```python
from build123d import *

# Parameters (mm, degrees)
STRUCTURAL_MEMBER1_DEPTH       = 1447.8
SKETCH12_R                     = 20.6375
CUT_EXTRUDE1_DEPTH             = 1451.304412873
F_1_2_0_5_DIAMETER_HOLE1_D     = 12.7
F_1_2_0_5_DIAMETER_HOLE1_DEPTH = 25.4
F_1_2_0_5_DIAMETER_HOLE1_TIP   = 3.815464931


with BuildPart() as part:
    # Sketch11 → Structural Member1 (new body)
    with BuildSketch(Plane(origin=(0, 0, 0), x_dir=(0, -1, 0), z_dir=(-1, 0, 0))):
        with BuildLine():
            Line((-25.4, -38.1), (25.4, -38.1))
            ThreePointArc((25.4, -38.1), (34.380256121, -34.380256121), (38.1, -25.4))
            Line((38.1, -25.4), (38.1, 25.4))
            ThreePointArc((38.1, 25.4), (34.380256121, 34.380256121), (25.4, 38.1))
            Line((25.4, 38.1), (-25.4, 38.1))
            ThreePointArc((-25.4, 38.1), (-34.380256121, 34.380256121), (-38.1, 25.4))
            Line((-38.1, 25.4), (-38.1, -25.4))
            ThreePointArc((-38.1, -25.4), (-34.380256121, -34.380256121), (-25.4, -38.1))
        make_face()
        with BuildLine():
            Line((-25.4, -34.925), (25.4, -34.925))
            ThreePointArc((25.4, -34.925), (32.135192091, -32.135192091), (34.925, -25.4))
            Line((34.925, -25.4), (34.925, 25.4))
            ThreePointArc((34.925, 25.4), (32.135192091, 32.135192091), (25.4, 34.925))
            Line((25.4, 34.925), (-25.4, 34.925))
            ThreePointArc((-25.4, 34.925), (-32.135192091, 32.135192091), (-34.925, 25.4))
            Line((-34.925, 25.4), (-34.925, -25.4))
            ThreePointArc((-34.925, -25.4), (-32.135192091, -32.135192091), (-25.4, -34.925))
        make_face(mode=Mode.SUBTRACT)
    extrude(amount=STRUCTURAL_MEMBER1_DEPTH)

    # Sketch12 → Cut-Extrude1 (cut, through all)
    with BuildSketch(Plane(origin=(0, 38.1, 0), x_dir=(1, 0, 0), z_dir=(0, 1, 0))):
        with Locations(Location((-723.9, 0, 0), (0, 0, 180))):
            Circle(SKETCH12_R)
    extrude(amount=-CUT_EXTRUDE1_DEPTH, mode=Mode.SUBTRACT)

    # 1/2 (0.5) Diameter Hole1
    with Locations(Plane(origin=(-800.1, 38.1, 0), x_dir=(0, 0, 1), z_dir=(0, 1, 0))):
        with Locations((0, 0), (0, 152.4)):
            Hole(F_1_2_0_5_DIAMETER_HOLE1_D / 2, depth=F_1_2_0_5_DIAMETER_HOLE1_DEPTH)
            with Locations((0, 0, -(F_1_2_0_5_DIAMETER_HOLE1_DEPTH + F_1_2_0_5_DIAMETER_HOLE1_TIP / 2))):  # 118° drill point
                Cone(0, F_1_2_0_5_DIAMETER_HOLE1_D / 2, F_1_2_0_5_DIAMETER_HOLE1_TIP, mode=Mode.SUBTRACT)


solid = part.part
```
Part model, mm, in its own coordinate system. A direction names the side the tool comes from. Round coordinates to 2 decimals unless told otherwise and drop trailing zeros. Loops run counter-clockwise (first coordinate to the right, second up) from the corner with the lowest first, then second, coordinate; pieces in that order, holes last.
1. Two-plate mould, pull along X, no slides. Class faces 1 (the face through (-1447.8, 0, -37)), 2 (the face through (0, 0, -37)), 3 (the face through (-714, 34.925, -22)), 4 (the face through (-703.282, 36.535, 0.907)): pulls with the +X half, pulls with the -X half, needs draft (parallel to the pull), parting line crosses it, or undercut.
Solutions:
face 1: pulls with the -X half
face 2: pulls with the +X half
face 3: needs draft
face 4: undercut
2. Drill centre lines: line 1 along Y through (x, z) = (-253.5, 13.5) (3 decimals); line 2 along Y through (x, z) = (-817, 33.5). Where is each one in solid material? Low to high.
Solutions:
line 1: y = -38.1 to -34.925, 34.925 to 38.1
line 2: y = -35.18 to -30.41, 30.41 to 35.18
3. Slice it at C-C (x = -236). Give the cut face in (y, z) (3 decimals), and give its area (3 significant figures).
Solutions:
outline: (-38.1, -25.4) arc R12.7 ccw to (-25.4, -38.1) - (25.4, -38.1) arc R12.7 ccw to (38.1, -25.4) - (38.1, 25.4) arc R12.7 ccw to (25.4, 38.1) - (-25.4, 38.1) arc R12.7 ccw to (-38.1, 25.4) - close; hole (-34.925, -25.4) arc R9.525 ccw to (-25.4, -34.925) - (25.4, -34.925) arc R9.525 ccw to (34.925, -25.4) - (34.925, 25.4) arc R9.525 ccw to (25.4, 34.925) - (-25.4, 34.925) arc R9.525 ccw to (-34.925, 25.4) - close
area: 867 mm2
4. 3-axis set-ups, long thin cutter, end or side, ignore diameter. For faces 5 (the face through (-714, 0, 38.1)), 6 (the face through (-714, 0, -34.925)): which of +Z, -Z, +X, -X, +Y, -Y reach the whole face in a straight line?
Solutions:
face 5: +Z, +X, -X, +Y, -Y
face 6: +X, -X
5. Flat gauge pins, fed straight in: pin 1 (12 mm diameter, centred on y = -18, z = -26.5, fed in from -X); pin 2 (11.5 mm diameter, centred on x = -800.1, z = 0, fed in from +Y) (3 decimals). Where does each tip first touch, or does it go through?
Solutions:
pin 1: passes through
pin 2: stops at y = -34.925
6. Slice it at B-B (y = 0.5). Give the cut face in (x, z) (3 decimals), and give its area (3 significant figures).
Solutions:
outline: (-1447.8, -38.1) - (0, -38.1) - (0, -34.925) - (-1447.8, -34.925) - close; (-1447.8, 34.925) - (0, 34.925) - (0, 38.1) - (-1447.8, 38.1) - close
area: 9,190 mm2
